Can you work these out from the drawing? Everything is in mm from the part's minimum corner. A direction names the side the tool comes from. Coordinates: 2 decimals unless noted, no trailing zeros. Loops run counter-clockwise (first coordinate to the right, second up) from the corner with the lowest first, then second, coordinate; pieces in that order, holes last. Notation, with made-up numbers: (-16.5, 0) -> (27.5, 0) arc R8 cw to (27.5, 5) -> close; hole circle Ø9 at (-13, 88). An arc over 180 degrees is marked (long way). Use one line per item in the form item = value. Start each with the question number.
(1) Thinking about a two-plate mould opening in X: for the marked faces 3, 4 and 5, which applies, released by +X, released by -X, zero draft, split by the parting line, or undercut?
(2) I'm going to push flat-ended pins straight in: pin 1 (2 mm diameter, centred on x = 58.5, z = 54.5, fed in from +Y); pin 2 (1 mm diameter, centred on x = 32.5, z = 49, fed in from -Y); pin 3 (3 mm diameter, centred on x = 8.5, z = 15, fed in from +Y); pin 4 (5 mm diameter, centred on y = 8, z = 22.5, fed in from +X). Where does each tip first touch, or does it pass through?
(3) Imagine slicing it at B-B (y = 6.25). List the corners of the cut face in (x, z) for me (1 decimal), plus the area to 3 significant figures.
(4) I need wall thicknesses on line 1 (X direction, y = 2, z = 26) (1 decimal); line 2 (Z direction, x = 21, y = 5); line 3 (X direction, y = 4, z = 46.5). Which ranges of each line are inside material? Lowest first, please. Write a range as [from, to].
(5) On a 3-axis mill with a long thin cutter (end or side, diameter ignored), from which of +Z, -Z, +X, -X, +Y, -Y can I reach the whole of each face in a straight line? I mean the marked faces 1 and 2. Say none if no direction works.
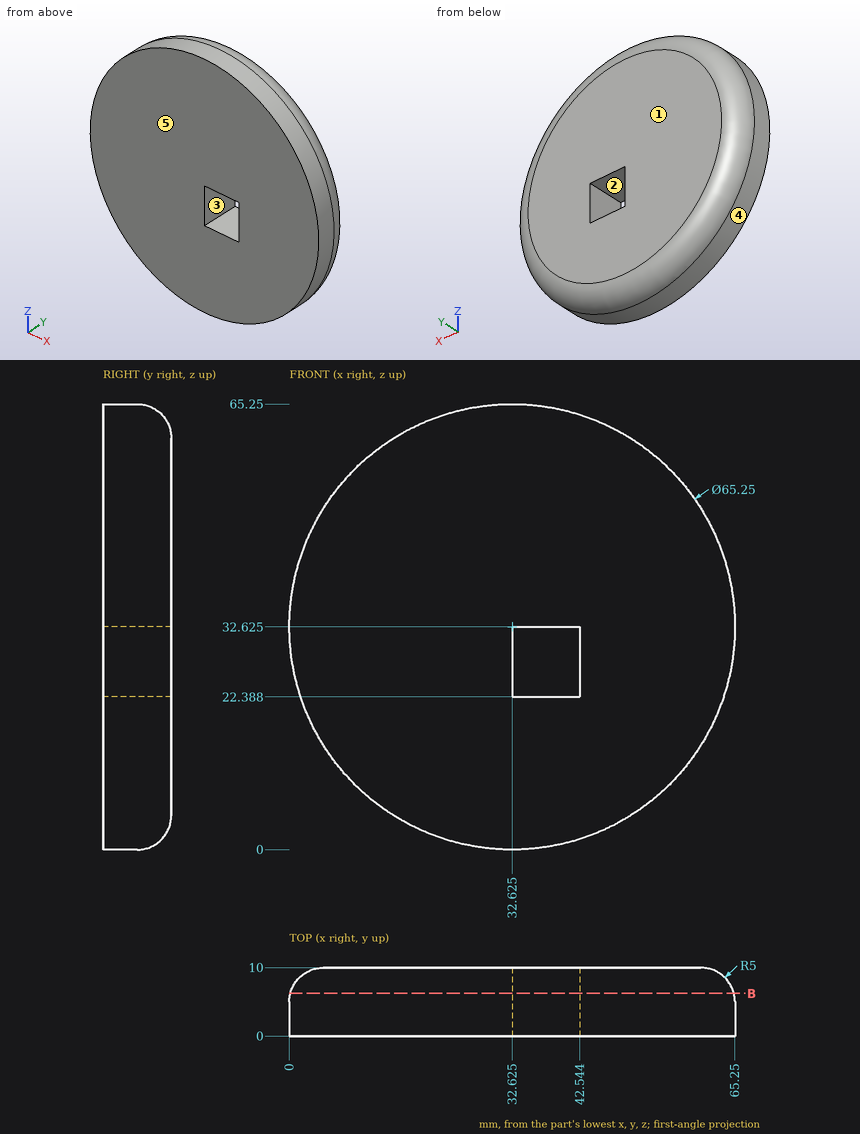
Worked out:
q1.face_3 = undercut
q1.face_4 = split by the parting line
q1.face_5 = zero draft
q2.pin_1 = through
q2.pin_2 = 0
q2.pin_3 = 9.94
q2.pin_4 = 64
q3.outline = circle Ø64.9 at (32.6, 32.6); hole (32.6, 22.4) -> (42.5, 22.4) -> (42.5, 32.6) -> (32.6, 32.6) -> close
q3.area = 3,210 mm2
q4.line_1 = [0.7, 32.6], [42.5, 64.6]
q4.line_2 = [2.14, 63.11]
q4.line_3 = [3.1, 62.15]
q5.face_1 = +Z, -Z, +X, -X, +Y
q5.face_2 = +Y, -Y
